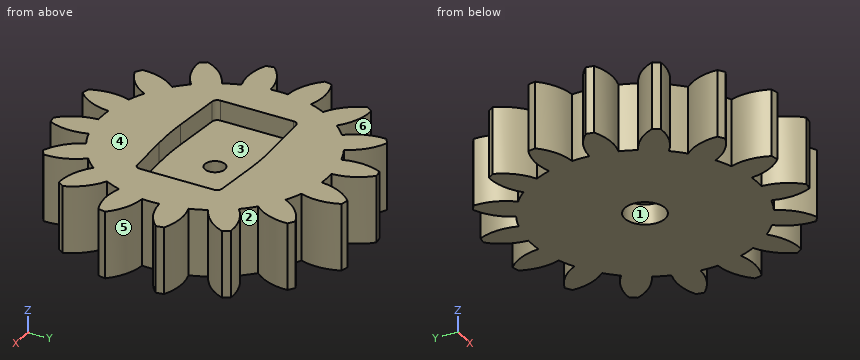
```python
from build123d import *

# Parameters (mm, degrees)
SALIENTE_EXTRUIR1_DEPTH = 5
CORTAR_EXTRUIR1_REACH   = 18.457
CROQUIS4_R              = 0.75
CORTAR_EXTRUIR2_START   = -3.5
CROQUIS4_3_R            = 1.5
CROQUIS4_3_R_2          = 0.75
CORTAR_EXTRUIR2_DEPTH   = 1.5
CROQUIS4_4_R            = 1.5
CROQUIS4_4_R_2          = 0.75
CORTAR_EXTRUIR3_DEPTH   = 1.5
REDONDEO2_R             = 0.4


with BuildPart() as part:
    # Croquis2 → Saliente-Extruir1 (new body)
    with BuildSketch(Plane.XY):
        with BuildLine():
            ThreePointArc((8.411340626, 0.651061533), (9.869549365, 1.023063112), (11.087096586, 1.907561087))
            ThreePointArc((11.087096586, 1.907561087), (11.033834405, 2.194766123), (10.973133635, 2.480491531))
            ThreePointArc((10.973133635, 2.480491531), (9.509783957, 2.831725957), (8.020215908, 2.617378277))
            ThreePointArc((8.020215908, 2.617378277), (7.794309676, 3.228508777), (7.521914983, 3.820383127))
            ThreePointArc((7.521914983, 3.820383127), (8.72676535, 4.722100097), (9.513149586, 6.005204821))
            ThreePointArc((9.513149586, 6.005204821), (9.354033138, 6.250165121), (9.188610559, 6.4909118))
            ThreePointArc((9.188610559, 6.4909118), (7.702240148, 6.255410419), (6.408086021, 5.487345971))
            ThreePointArc((6.408086021, 5.487345971), (5.965506359, 5.965506359), (5.487345971, 6.408086021))
            ThreePointArc((5.487345971, 6.408086021), (6.255410419, 7.702240148), (6.4909118, 9.188610559))
            ThreePointArc((6.4909118, 9.188610559), (6.250165121, 9.354033138), (6.005204821, 9.513149586))
            ThreePointArc((6.005204821, 9.513149586), (4.722100097, 8.72676535), (3.820383127, 7.521914983))
            ThreePointArc((3.820383127, 7.521914983), (3.228508777, 7.794309676), (2.617378277, 8.020215908))
            ThreePointArc((2.617378277, 8.020215908), (2.831725957, 9.509783957), (2.480491531, 10.973133635))
            ThreePointArc((2.480491531, 10.973133635), (2.194766123, 11.033834405), (1.907561087, 11.087096586))
            ThreePointArc((1.907561087, 11.087096586), (1.023063112, 9.869549365), (0.651061533, 8.411340626))
            ThreePointArc((0.651061533, 8.411340626), (0, 8.4365), (-0.651061533, 8.411340626))
            ThreePointArc((-0.651061533, 8.411340626), (-1.023063112, 9.869549365), (-1.907561087, 11.087096586))
            ThreePointArc((-1.907561087, 11.087096586), (-2.194766123, 11.033834405), (-2.480491531, 10.973133635))
            ThreePointArc((-2.480491531, 10.973133635), (-2.831725957, 9.509783957), (-2.617378277, 8.020215908))
            ThreePointArc((-2.617378277, 8.020215908), (-3.228508777, 7.794309676), (-3.820383127, 7.521914983))
            ThreePointArc((-3.820383127, 7.521914983), (-4.722100097, 8.72676535), (-6.005204821, 9.513149586))
            ThreePointArc((-6.005204821, 9.513149586), (-6.250165121, 9.354033138), (-6.4909118, 9.188610559))
            ThreePointArc((-6.4909118, 9.188610559), (-6.255410419, 7.702240148), (-5.487345971, 6.408086021))
            ThreePointArc((-5.487345971, 6.408086021), (-5.965506359, 5.965506359), (-6.408086021, 5.487345971))
            ThreePointArc((-6.408086021, 5.487345971), (-7.702240148, 6.255410419), (-9.188610559, 6.4909118))
            ThreePointArc((-9.188610559, 6.4909118), (-9.354033138, 6.250165121), (-9.513149586, 6.005204821))
            ThreePointArc((-9.513149586, 6.005204821), (-8.72676535, 4.722100097), (-7.521914983, 3.820383127))
            ThreePointArc((-7.521914983, 3.820383127), (-7.794309676, 3.228508777), (-8.020215908, 2.617378277))
            ThreePointArc((-8.020215908, 2.617378277), (-9.509783957, 2.831725957), (-10.973133635, 2.480491531))
            ThreePointArc((-10.973133635, 2.480491531), (-11.033834405, 2.194766123), (-11.087096586, 1.907561087))
            ThreePointArc((-11.087096586, 1.907561087), (-9.869549365, 1.023063112), (-8.411340626, 0.651061533))
            ThreePointArc((-8.411340626, 0.651061533), (-8.4365, 0), (-8.411340626, -0.651061533))
            ThreePointArc((-8.411340626, -0.651061533), (-9.869549365, -1.023063112), (-11.087096586, -1.907561087))
            ThreePointArc((-11.087096586, -1.907561087), (-11.033834405, -2.194766123), (-10.973133635, -2.480491531))
            ThreePointArc((-10.973133635, -2.480491531), (-9.509783957, -2.831725957), (-8.020215908, -2.617378277))
            ThreePointArc((-8.020215908, -2.617378277), (-7.794309676, -3.228508777), (-7.521914983, -3.820383127))
            ThreePointArc((-7.521914983, -3.820383127), (-8.72676535, -4.722100097), (-9.513149586, -6.005204821))
            ThreePointArc((-9.513149586, -6.005204821), (-9.354033138, -6.250165121), (-9.188610559, -6.4909118))
            ThreePointArc((-9.188610559, -6.4909118), (-7.702240148, -6.255410419), (-6.408086021, -5.487345971))
            ThreePointArc((-6.408086021, -5.487345971), (-5.965506359, -5.965506359), (-5.487345971, -6.408086021))
            ThreePointArc((-5.487345971, -6.408086021), (-6.255410419, -7.702240148), (-6.4909118, -9.188610559))
            ThreePointArc((-6.4909118, -9.188610559), (-6.250165121, -9.354033138), (-6.005204821, -9.513149586))
            ThreePointArc((-6.005204821, -9.513149586), (-4.722100097, -8.72676535), (-3.820383127, -7.521914983))
            ThreePointArc((-3.820383127, -7.521914983), (-3.228508777, -7.794309676), (-2.617378277, -8.020215908))
            ThreePointArc((-2.617378277, -8.020215908), (-2.831725957, -9.509783957), (-2.480491531, -10.973133635))
            ThreePointArc((-2.480491531, -10.973133635), (-2.194766123, -11.033834405), (-1.907561087, -11.087096586))
            ThreePointArc((-1.907561087, -11.087096586), (-1.023063112, -9.869549365), (-0.651061533, -8.411340626))
            ThreePointArc((-0.651061533, -8.411340626), (0, -8.4365), (0.651061533, -8.411340626))
            ThreePointArc((0.651061533, -8.411340626), (1.023063112, -9.869549365), (1.907561087, -11.087096586))
            ThreePointArc((1.907561087, -11.087096586), (2.194766123, -11.033834405), (2.480491531, -10.973133635))
            ThreePointArc((2.480491531, -10.973133635), (2.831725957, -9.509783957), (2.617378277, -8.020215908))
            ThreePointArc((2.617378277, -8.020215908), (3.228508777, -7.794309676), (3.820383127, -7.521914983))
            ThreePointArc((3.820383127, -7.521914983), (4.722100097, -8.72676535), (6.005204821, -9.513149586))
            ThreePointArc((6.005204821, -9.513149586), (6.250165121, -9.354033138), (6.4909118, -9.188610559))
            ThreePointArc((6.4909118, -9.188610559), (6.255410419, -7.702240148), (5.487345971, -6.408086021))
            ThreePointArc((5.487345971, -6.408086021), (5.965506359, -5.965506359), (6.408086021, -5.487345971))
            ThreePointArc((6.408086021, -5.487345971), (7.702240148, -6.255410419), (9.188610559, -6.4909118))
            ThreePointArc((9.188610559, -6.4909118), (9.354033138, -6.250165121), (9.513149586, -6.005204821))
            ThreePointArc((9.513149586, -6.005204821), (8.72676535, -4.722100097), (7.521914983, -3.820383127))
            ThreePointArc((7.521914983, -3.820383127), (7.794309676, -3.228508777), (8.020215908, -2.617378277))
            ThreePointArc((8.020215908, -2.617378277), (9.509783957, -2.831725957), (10.973133635, -2.480491531))
            ThreePointArc((10.973133635, -2.480491531), (11.033834405, -2.194766123), (11.087096586, -1.907561087))
            ThreePointArc((11.087096586, -1.907561087), (9.869549365, -1.023063112), (8.411340626, -0.651061533))
            ThreePointArc((8.411340626, -0.651061533), (8.4365, 0), (8.411340626, 0.651061533))
        make_face()
    extrude(amount=SALIENTE_EXTRUIR1_DEPTH)

    # Croquis4 → Cortar-Extruir1 (cut, up to next)
    with BuildSketch(Plane.XY.offset(5), mode=Mode.PRIVATE) as cortar_extruir1_sk1:
        Circle(CROQUIS4_R)
    cortar_extruir1_tool1 = extrude(cortar_extruir1_sk1.sketch, amount=-CORTAR_EXTRUIR1_REACH, mode=Mode.PRIVATE) & part.part
    add(cortar_extruir1_tool1.solids().sort_by_distance((0, 0, 5))[0], mode=Mode.SUBTRACT)

    # Croquis4<3> → Cortar-Extruir2 (cut)
    with BuildSketch(Plane.XY.offset(5).offset(CORTAR_EXTRUIR2_START)):
        Circle(CROQUIS4_3_R)
        Circle(CROQUIS4_3_R_2, mode=Mode.SUBTRACT)
    extrude(amount=-CORTAR_EXTRUIR2_DEPTH, mode=Mode.SUBTRACT)

    # Croquis4<4> → Cortar-Extruir3 (cut)
    # profile 1 of 2: a face of its own
    with BuildSketch(Plane.XY.offset(5)):
        with BuildLine():
            Line((-5.5, 3.135446053), (-5.5, -3.135446053))
            Line((-5.5, -3.135446053), (-1.395129475, -3.422486562))
            ThreePointArc((-1.395129475, -3.422486562), (0, -3.471205557), (1.395129475, -3.422486562))
            Line((1.395129475, -3.422486562), (5, -3.170409459))
            Line((5, -3.170409459), (5, 3.170409459))
            Line((5, 3.170409459), (1.395129475, 3.422486562))
            ThreePointArc((1.395129475, 3.422486562), (0, 3.471205557), (-1.395129475, 3.422486562))
            Line((-1.395129475, 3.422486562), (-5.5, 3.135446053))
        make_face()
        Circle(CROQUIS4_4_R, mode=Mode.SUBTRACT)
    # profile 2 of 2: a face of its own
    with BuildSketch(Plane.XY.offset(5)):
        Circle(CROQUIS4_4_R)
        Circle(CROQUIS4_4_R_2, mode=Mode.SUBTRACT)
    extrude(amount=-CORTAR_EXTRUIR3_DEPTH, mode=Mode.SUBTRACT)

    # Redondeo2
    redondeo2_edges = [part.edges().sort_by_distance(p)[0] for p in [
        (5, 3.170409459, 4.25),
        (5, -3.170409459, 4.25),
        (-5.5, -3.135446053, 4.25),
        (-5.5, 3.135446053, 4.25),
    ]]
    fillet(redondeo2_edges, radius=REDONDEO2_R)


solid = part.part
```
Verification items for the finished model (mm, model axes). Face numbers are marked on the shaded views. A direction names the side the tool comes from. Give positions to 0.01 mm unless a question says otherwise; leave off trailing zeros. Loops run counter-clockwise (first coordinate to the right, second up) from the corner with the lowest first, then second, coordinate; pieces in that order, holes last. Notation, with made-up numbers: M -40,2.5 L -2,2.5 A28 ccw -2,32.5 Z; hole C 45.25,-37.75 d11. An arc over 180 degrees is marked long. Return JSON: item names as keys, results as strings.
1) Material ranges on L1, parallel to Y at x = -6, z = 1.3; L2, parallel to X at y = -7.75, z = 1.85; L3, parallel to Z at x = -1.5, y = 3.25, recorded low to high. Write a range as [from, to].
Findings:
{"L1": "y = [-9.51, -7.14], [-5.93, 5.93], [7.14, 9.51]", "L2": "x = [-6.27, -3.94], [-3.33, 3.33], [3.94, 6.27]", "L3": "z = [0, 3.5]"}
2) Gauge pin test, flat ends, axial feed: P1, Ø12, axis at x = -6.5, y = 6, coming from the -Z side; P2, Ø1.4, axis at x = 0, y = 0, coming from the -Z side; P3, Ø0.8, axis at y = -1, z = 4.5, coming from the -X side; P4, Ø2, axis at x = 2.5, y = 1, coming from the +Z side. Record the tip position at first contact, or that the pin passes through.
Findings:
{"P1": "stops at z = 0", "P2": "passes through", "P3": "stops at x = -10.51", "P4": "stops at z = 3.5"}
3) Section check C-C, the plane y = 5. Enter the section's corners in (x, z), and give its area (3 significant figures).
Findings:
{"outline": "M -8.96,0 L 8.96,0 L 8.96,5 L -8.96,5 Z", "area": "89.6 mm2"}
4) Tool access check on the marked faces 1, 2 and 3. Record the directions out of +Z, -Z, +X, -X, +Y, -Y that give a thin tool (end or side, any length) a straight path to the whole face; none if there is none.
Findings:
{"face 1": "-Z", "face 2": "+Z, -Z", "face 3": "+Z"}
5) Section check A-A, the plane x = 0. Enter the section's corners in (y, z), and give its area (3 significant figures).
Findings:
{"outline": "M -8.44,0 L -1.5,0 L -1.5,1.5 L -0.75,1.5 L -0.75,3.5 L -3.47,3.5 L -3.47,5 L -8.44,5 Z; M 0.75,1.5 L 1.5,1.5 L 1.5,0 L 8.44,0 L 8.44,5 L 3.47,5 L 3.47,3.5 L 0.75,3.5 Z", "area": "66.5 mm2"}
6) Section check B-B, the plane y = 0. Enter the section's corners in (x, z).
Findings:
{"outline": "M -8.44,0 L -1.5,0 L -1.5,1.5 L -0.75,1.5 L -0.75,3.5 L -5.5,3.5 L -5.5,5 L -8.44,5 Z; M 0.75,1.5 L 1.5,1.5 L 1.5,0 L 8.44,0 L 8.44,5 L 5,5 L 5,3.5 L 0.75,3.5 Z"}
7) Mould release check, pull along X, two halves, no side actions. Record for the marked faces 4, 5 and 6: released by +X, released by -X, zero draft, split by the parting line, or undercut.
Findings:
{"face 4": "zero draft", "face 5": "released by +X", "face 6": "undercut"}
8) Section check D-D, the plane y = -4.5. Enter the section's corners in (x, z).
Findings:
{"outline": "M -8.51,0 L 8.51,0 L 8.51,5 L -8.51,5 Z"}
